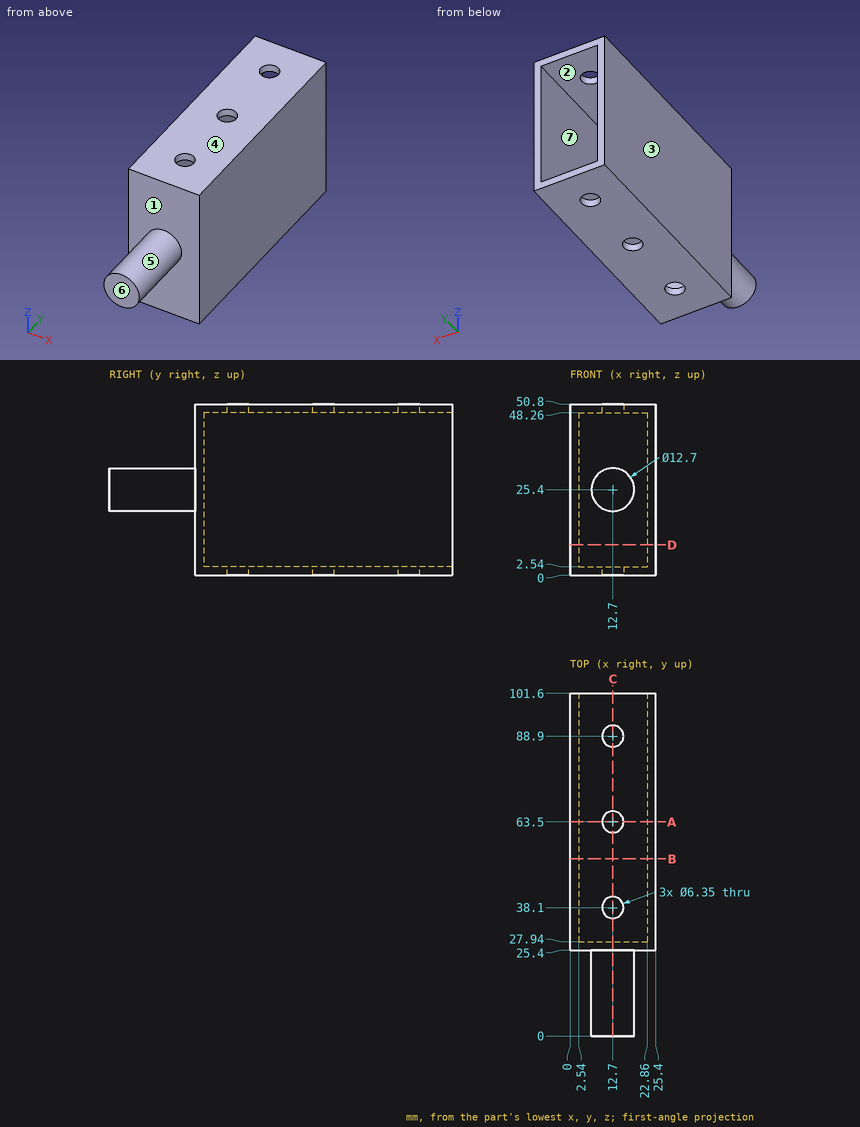
Design review of the part shown in the three views and the two pictorial views. Dimensions are in mm from the part's minimum x, y and z. A direction names the side the tool comes from. Round coordinates to 2 decimals unless told otherwise and drop trailing zeros. Write each loop counter-clockwise with the first axis right and the second up, starting at its lowest first coordinate (ties: lowest second). Pieces come first, ordered by that corner, then holes.
Item 1: For the marked faces 1, 2 and 3, list the 3-axis set-ups (+Z, -Z, +X, -X, +Y, -Y) from which the entire face can be reached by the end or side of a thin tool; tool diameter is ignored.
Item 2: We need section C-C on x = 12.7. State how many separate pieces and enclosed holes the cut face has, and give its area (3 significant figures).
Item 3: We need section A-A on y = 63.5. Write out the cut boundary in (x, z) (3 decimals).
Item 4: We need section D-D on z = 9. Write out the cut boundary in (x, y).
Item 5: For probe 1 along Y at (x, z) = (12.7, 1.6) (3 decimals); probe 2 along X at (y, z) = (50, 46); probe 3 along Z at (x, y) = (19.75, 93), list the stretches that pass through material, from the lowest coordinate up.
Item 6: We need section B-B on y = 52.5. Write out the cut boundary in (x, z), and give its area (3 significant figures).
Item 7: The part is to be moulded in two halves that separate along Z. For the marked faces 4, 5, 6 and 7, say which applies: +Z half, -Z half, draft (parallel to the pull), parting line (faces both ways), or undercut.
Returned:
1. face 1: -Y
1. face 2: +Y
1. face 3: +Z, -Z, -X, +Y, -Y
2. separate pieces: 7
2. enclosed holes: 0
2. area: 729 mm2
3. outline: (0, 0) - (9.525, 0) - (9.525, 2.54) - (2.54, 2.54) - (2.54, 48.26) - (9.525, 48.26) - (9.525, 50.8) - (0, 50.8) - close; (15.875, 0) - (25.4, 0) - (25.4, 50.8) - (15.875, 50.8) - (15.875, 48.26) - (22.86, 48.26) - (22.86, 2.54) - (15.875, 2.54) - close
4. outline: (0, 25.4) - (25.4, 25.4) - (25.4, 101.6) - (22.86, 101.6) - (22.86, 27.94) - (2.54, 27.94) - (2.54, 101.6) - (0, 101.6) - close
5. probe 1: y = 25.4 to 34.925, 41.275 to 60.325, 66.675 to 85.725, 92.075 to 101.6
5. probe 2: x = 0 to 2.54, 22.86 to 25.4
5. probe 3: z = 0 to 2.54, 48.26 to 50.8
6. outline: (0, 0) - (25.4, 0) - (25.4, 50.8) - (0, 50.8) - close; hole (2.54, 2.54) - (22.86, 2.54) - (22.86, 48.26) - (2.54, 48.26) - close
6. area: 361 mm2
7. face 4: +Z half
7. face 5: parting line
7. face 6: draft
7. face 7: undercut
